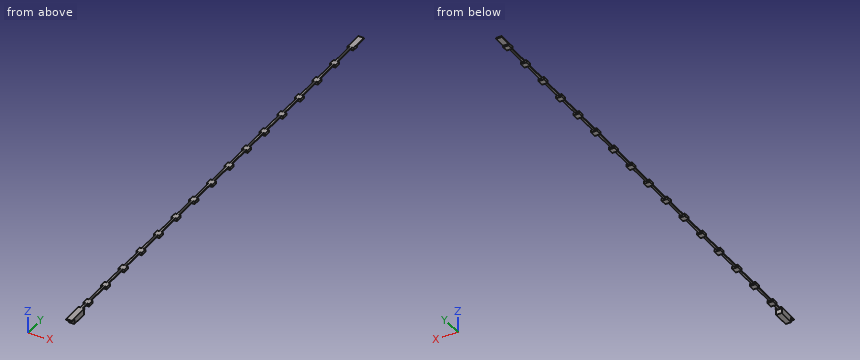
from build123d import *

# Parameters (mm, degrees)
SKETCH2_W           = 5.58
SKETCH2_H           = 21.51
BOSS_EXTRUDE1_DEPTH = 0.5
BOSS_EXTRUDE2_DEPTH = 0.5
SKETCH4_W           = 5.58
SKETCH4_H           = 6
BOSS_EXTRUDE3_DEPTH = 2.6
LPATTERN1_COUNT     = 16
LPATTERN1_PITCH     = 30
SKETCH5_W           = 5.58
SKETCH5_H           = 1
BOSS_EXTRUDE4_DEPTH = 12
SKETCH9_W           = 5.58
SKETCH9_H           = 16
BOSS_EXTRUDE6_DEPTH = 5


with BuildPart() as part:
    # Sketch2 → Boss-Extrude1 (new body, symmetric)
    with BuildSketch(Plane.XY):
        with Locations((0, 10.755)):
            Rectangle(SKETCH2_W, SKETCH2_H)
    extrude(amount=BOSS_EXTRUDE1_DEPTH, both=True)

    # Sketch3 → Boss-Extrude2 (add, symmetric)
    with BuildSketch(Plane.XY):
        Polygon((-2.79, 35.51), (2.79, 35.51), (2.79, 29.51), (1, 29.51), (1, 4.51), (-1, 4.51), (-1, 29.51), (-2.79, 29.51), align=None)
    boss_extrude2 = extrude(amount=BOSS_EXTRUDE2_DEPTH, both=True)

    # Sketch4 → Boss-Extrude3 (add)
    with BuildSketch(Plane.XY.offset(0.5)):
        with Locations((0, 32.51)):
            Rectangle(SKETCH4_W, SKETCH4_H)
    boss_extrude3 = extrude(amount=-BOSS_EXTRUDE3_DEPTH)

    # LPattern1: Boss-Extrude2, Boss-Extrude3 ×16
    with Locations(*[(0, i * LPATTERN1_PITCH, 0) for i in range(1, LPATTERN1_COUNT)]):
        add(boss_extrude2)
        add(boss_extrude3)

    # Sketch5 → Boss-Extrude4 (add)
    with BuildSketch(Plane(origin=(0, 485.51, 0), x_dir=(1, 0, 0), z_dir=(0, 1, 0))):
        Rectangle(SKETCH5_W, SKETCH5_H)
    extrude(amount=BOSS_EXTRUDE4_DEPTH)

    # Sketch9 → Boss-Extrude6 (add)
    with BuildSketch(Plane.XY.offset(-0.5)):
        with Locations((0, 12.61)):
            Rectangle(SKETCH9_W, SKETCH9_H)
    extrude(amount=-BOSS_EXTRUDE6_DEPTH)


solid = part.part
Check sheet for the modelled part. Datum: model origin and axes. Units: mm. Round coordinates to 2 decimals unless told otherwise and drop trailing zeros. Order: outer loops, then holes, each group sorted by start corner. A loop starts at its lowest first (then second) coordinate and runs counter-clockwise, first axis right, second up.
Q1. Cross-section at A-A, the plane y = 135. Enter the section's corners in (x, z), plus the area to 3 significant figures.
Filled sheet:
outline: (-1, -0.5) - (1, -0.5) - (1, 0.5) - (-1, 0.5) - close
area: 2.00 mm2
Q2. Depth check by flat-ended pin: P1, Ø0.8, axis at y = 45.5, z = 0, coming from the +X side; P2, Ø3, axis at x = 1, y = 331.5, coming from the -Z side; P3, Ø0.8, axis at y = 288.5, z = 0, coming from the -X side. Enter the tip coordinate at first touch or a pass-through.
Filled sheet:
P1: stops at x = 1
P2: stops at z = -2.1
P3: stops at x = -1
Q3. Scan lines: L1, parallel to Y at x = -0.25, z = -5.2; L2, parallel to Z at x = -0.2, y = 368.5; L3, parallel to Z at x = -1, y = 302. Record each from-to range of solid material in increasing order.
Filled sheet:
L1: y = 4.61 to 20.61
L2: z = -0.5 to 0.5
L3: z = -2.1 to 0.5
Q4. Cross-section at B-B, the plane z = -3.3. Enter the section's corners in (x, y), plus the area to 3 significant figures.
Filled sheet:
outline: (-2.79, 4.61) - (2.79, 4.61) - (2.79, 20.61) - (-2.79, 20.61) - close
area: 89.3 mm2
